Build history of the part. All positions in model axes, mm. A direction names the side the tool comes from. Coordinates: 2 decimals unless noted, no trailing zeros. Write each loop counter-clockwise with the first axis right and the second up, starting at its lowest first coordinate (ties: lowest second). Pieces come first, ordered by that corner, then holes.
from build123d import *
from build123d import SkipClean  # not in build123d's __all__

# Parameters (mm, degrees)
F1_DEPTH = 50
F2_DEPTH = 5
F4_DEPTH = 5
F5_W     = 30
F5_H     = 30
F6_DEPTH = 10
F7_W     = 30
F7_H     = 20.1446080953
F8_DEPTH = 15


with BuildPart() as f1:
    # F0 (on Front) → F1 (new body)
    with BuildSketch(Plane.XZ):
        with BuildLine():
            Line((-34.2131151259, 22.4876786768), (-44.2131151259, 22.4876786768))
            Line((-44.2131151259, 22.4876786768), (-49.2131151259, 17.4876786768))
            Line((-49.2131151259, 17.4876786768), (-49.2131151259, -7.5123213232))
            ThreePointArc((-49.2131151259, -7.5123213232), (-31.5354455962, -14.8346517935), (-24.2131151259, -32.5123213232))
            Line((-24.2131151259, -32.5123213232), (15.7868848741, -32.5123213232))
            ThreePointArc((15.7868848741, -32.5123213232), (23.1092153444, -14.8346517935), (40.7868848741, -7.5123213232))
            Line((40.7868848741, -7.5123213232), (40.7868848741, 2.4876786768))
            Line((40.7868848741, 2.4876786768), (-19.2131151259, 2.4876786768))
            Line((-19.2131151259, 2.4876786768), (-19.2131151259, 7.4876786768))
            Line((-19.2131151259, 7.4876786768), (-34.2131151259, 22.4876786768))
        make_face()
        with BuildLine():
            Line((-49.2131151259, -17.5123213232), (-49.2131151259, -7.5123213232))
            ThreePointArc((-49.2131151259, -7.5123213232), (-66.8907846556, -50.1899908528), (-24.2131151259, -32.5123213232))
            Line((-24.2131151259, -32.5123213232), (-34.2131151259, -32.5123213232))
            ThreePointArc((-34.2131151259, -32.5123213232), (-59.8197168437, -43.118923041), (-49.2131151259, -17.5123213232))
        make_face()
        with BuildLine():
            ThreePointArc((-24.2131151259, -32.5123213232), (-31.5354455962, -14.8346517935), (-49.2131151259, -7.5123213232))
            Line((-49.2131151259, -7.5123213232), (-49.2131151259, -17.5123213232))
            ThreePointArc((-49.2131151259, -17.5123213232), (-38.6065134081, -21.9057196054), (-34.2131151259, -32.5123213232))
            Line((-34.2131151259, -32.5123213232), (-24.2131151259, -32.5123213232))
        make_face()
        with BuildLine():
            ThreePointArc((40.7868848741, -7.5123213232), (23.1092153444, -14.8346517935), (15.7868848741, -32.5123213232))
            Line((15.7868848741, -32.5123213232), (25.7868848741, -32.5123213232))
            ThreePointArc((25.7868848741, -32.5123213232), (30.1802831563, -21.9057196054), (40.7868848741, -17.5123213232))
            Line((40.7868848741, -17.5123213232), (40.7868848741, -7.5123213232))
        make_face()
        with BuildLine():
            Line((25.7868848741, -32.5123213232), (15.7868848741, -32.5123213232))
            ThreePointArc((15.7868848741, -32.5123213232), (40.7868848741, -57.5123213232), (65.7868848741, -32.5123213232))
            ThreePointArc((65.7868848741, -32.5123213232), (58.4645544038, -14.8346517935), (40.7868848741, -7.5123213232))
            Line((40.7868848741, -7.5123213232), (40.7868848741, -17.5123213232))
            ThreePointArc((40.7868848741, -17.5123213232), (51.3934865919, -21.9057196054), (55.7868848741, -32.5123213232))
            ThreePointArc((55.7868848741, -32.5123213232), (40.7868848741, -47.5123213232), (25.7868848741, -32.5123213232))
        make_face()
    extrude(amount=F1_DEPTH)

    # F0 (on Front) → F2 (cut)
    with BuildSketch(Plane.XZ):
        with BuildLine():
            Line((-34.2131151259, 22.4876786768), (-44.2131151259, 22.4876786768))
            Line((-44.2131151259, 22.4876786768), (-49.2131151259, 17.4876786768))
            Line((-49.2131151259, 17.4876786768), (-49.2131151259, -7.5123213232))
            ThreePointArc((-49.2131151259, -7.5123213232), (-31.5354455962, -14.8346517935), (-24.2131151259, -32.5123213232))
            Line((-24.2131151259, -32.5123213232), (15.7868848741, -32.5123213232))
            ThreePointArc((15.7868848741, -32.5123213232), (23.1092153444, -14.8346517935), (40.7868848741, -7.5123213232))
            Line((40.7868848741, -7.5123213232), (40.7868848741, 2.4876786768))
            Line((40.7868848741, 2.4876786768), (-19.2131151259, 2.4876786768))
            Line((-19.2131151259, 2.4876786768), (-19.2131151259, 7.4876786768))
            Line((-19.2131151259, 7.4876786768), (-34.2131151259, 22.4876786768))
        make_face()
    extrude(amount=F2_DEPTH, mode=Mode.SUBTRACT)

    # F3 (on face) → F4 (cut)
    with BuildSketch(Plane.XZ.offset(50)):
        with BuildLine():
            Line((-34.2131151259, 22.4876786768), (-44.2131151259, 22.4876786768))
            Line((-44.2131151259, 22.4876786768), (-49.2131151259, 17.4876786768))
            Line((-49.2131151259, 17.4876786768), (-49.2131151259, -7.5123213232))
            ThreePointArc((-49.2131151259, -7.5123213232), (-31.5354455962, -14.8346517935), (-24.2131151259, -32.5123213232))
            Line((-24.2131151259, -32.5123213232), (15.7868848741, -32.5123213232))
            ThreePointArc((15.7868848741, -32.5123213232), (23.1092153444, -14.8346517935), (40.7868848741, -7.5123213232))
            Line((40.7868848741, -7.5123213232), (40.7868848741, 2.4876786768))
            Line((40.7868848741, 2.4876786768), (-19.2131151259, 2.4876786768))
            Line((-19.2131151259, 2.4876786768), (-19.2131151259, 7.4876786768))
            Line((-19.2131151259, 7.4876786768), (-34.2131151259, 22.4876786768))
        make_face()
    with SkipClean():  # cleaning this boolean's faces spoils the solid; the shape is the same uncleaned
        extrude(amount=-F4_DEPTH, mode=Mode.SUBTRACT)

    # F5 (on face) → F6 (cut)
    with BuildSketch(Plane.XY.offset(2.4876786768)):
        with Locations((-4.2131151259, -25)):
            Rectangle(F5_W, F5_H)
    extrude(amount=-F6_DEPTH, mode=Mode.SUBTRACT)

    # F7 (on face) → F8 (cut)
    with BuildSketch(Plane.YZ.offset(-19.2131151259)):
        Polygon((-40, 2.4876786768), (-40, -7.5123213232), (-10, -7.5123213232), (-10, 2.4876786768), (-10, 7.4876786768), (-40, 7.4876786768), align=None)
        with Locations((-25, 17.5599827245)):
            Rectangle(F7_W, F7_H)
    extrude(amount=-F8_DEPTH, mode=Mode.SUBTRACT)


solid = f1.part
(1) 3-axis set-ups, long thin cutter, end or side, ignore diameter. For faces 4 (the flat face through (-11, -25, -7.512)), 5 (the flat face through (-19.213, -42, 5)), 6 (the flat face through (-38, 0, -43)), 7 (the flat face through (-4, -25, -32.512)), 8 (the flat face through (-5, -5, -5)): which of +Z, -Z, +X, -X, +Y, -Y reach the whole face in a straight line?
(2) Slice it at D-D, the plane z = -42. List the corners of the cut face in (x, y).
(3) Slice it at A-A, the plane y = -7. List the corners of the cut face in (x, z), and give its area (3 significant figures).
(4) Slice it at B-B, the plane x = 48. List the corners of the cut face in (y, z), and give its area (3 significant figures).
(5) Two-plate mould, pull along X, no slides. Class faces 1 (the flat face through (-49.213, -25, 5)), 2 (the flat face through (-19.213, -7, 5)), 3 (the flat face through (-34.213, -25, 8)): pulls with the +X half, pulls with the -X half, needs draft (parallel to the pull), parting line crosses it, or undercut.
(6) Slice it at C-C, the plane z = -26. List the corners of the cut face in (x, y).
(7) Probe L1, parallel to X at y = -27.5, z = -4; L2, parallel to X at y = -19.5, z = -31; L3, parallel to X at y = -23, z = -43. List the from-to ranges inside material, lowest first.
(8) Flat gauge pins, fed straight in: P1, Ø11, axis at y = -29, z = -4.5, coming from the -X side; P2, Ø3, axis at y = -44, z = 10, coming from the -X side; P3, Ø12, axis at x = -9, y = -9, coming from the +Z side. Where does each tip first touch, or does it go through?
Results:
1. face 4: +Z
1. face 5: +Z, +X, +Y, -Y
1. face 6: +Z, -Z, +X, -X, +Y
1. face 7: -Z, +Y, -Y
1. face 8: +Z, +Y
2. outline: (-72.34, -50) - (-60.83, -50) - (-60.83, 0) - (-72.34, 0) - close; (-37.59, -50) - (-26.08, -50) - (-26.08, 0) - (-37.59, 0) - close; (17.66, -50) - (29.17, -50) - (29.17, 0) - (17.66, 0) - close; (52.41, -50) - (63.92, -50) - (63.92, 0) - (52.41, 0) - close
3. outline: (-49.21, -7.51) arc R25 ccw (long way) to (-24.21, -32.51) - (15.79, -32.51) arc R25 ccw (long way) to (40.79, -7.51) - (40.79, 2.49) - (-19.21, 2.49) - (-19.21, 7.49) - (-34.21, 22.49) - (-44.21, 22.49) - (-49.21, 17.49) - close; hole circle Ø30 at (-49.21, -32.51); hole circle Ø30 at (40.79, -32.51)
3. area: 5,160 mm2
4. outline: (-50, -56.45) - (0, -56.45) - (0, -45.66) - (-50, -45.66) - close; (-50, -19.36) - (0, -19.36) - (0, -8.58) - (-50, -8.58) - close
4. area: 1,080 mm2
5. face 1: pulls with the -X half
5. face 2: pulls with the +X half
5. face 3: undercut
6. outline: (-73.35, -50) - (-62.73, -50) - (-62.73, 0) - (-73.35, 0) - close; (-35.7, -50) - (-25.08, -50) - (-25.08, -45) - (16.65, -45) - (16.65, -50) - (27.27, -50) - (27.27, 0) - (16.65, 0) - (16.65, -5) - (-25.08, -5) - (-25.08, 0) - (-35.7, 0) - close; (54.3, -50) - (64.92, -50) - (64.92, 0) - (54.3, 0) - close
7. L1: x = -49.21 to -34.21, 10.79 to 40.79
7. L2: x = -74.17 to -64.14, -34.29 to 25.86, 55.71 to 65.74
7. L3: x = -71.91 to -59.94, -38.49 to -26.52, 18.09 to 30.06, 51.51 to 63.48
8. P1: stops at x = -60.08
8. P2: stops at x = -49.21
8. P3: stops at z = 2.49
